```python
from build123d import *

# Parameters (mm, degrees)
F2_R     = 4.064
F3_DEPTH = 12.7
F3_TAPER = 1
F5_DEPTH = 0.79375
F6_COUNT = 8


with BuildPart() as f1:
    # F0 (on Front) → F1 (revolve)
    with BuildSketch(Plane.XZ):
        Polygon((-6.35, 0), (0, 0), (0, 22.9133968065), (-3.175, 22.9133968065), (-3.175, 16.5633968065), (-6.35, 9.525), align=None)
    revolve(axis=Axis((0, 0, 20.1071155777), (0, 0, 1)))

    # F2 (on face) → F3 (join)
    with BuildSketch(Plane(origin=(0, 0, 0), x_dir=(1, 0, 0), z_dir=(0, 0, -1))):
        Circle(F2_R)
    extrude(amount=F3_DEPTH, taper=F3_TAPER)

    # F4 (on Front) → F5 (join, symmetric)
    with BuildSketch(Plane.XZ):
        Polygon((-18.3153760806, 1.7450850807), (-6.35, 0), (-6.0325, 0), (-6.0325, 9.4567020336), (-2.8575, 16.4950988401), (-2.8575, 22.9133968065), (-3.175, 22.9133968065), (-6.35, 22.9133968065), (-38.1, 28.0183404684), (-12.5059876591, 9.994440712), align=None)
    extrude(amount=F5_DEPTH, both=True)

    # F6: F1 ×8 about axis
    f6_axis = Axis((0, 0, 20.1071155777), (0, 0, 1))


with BuildPart() as f1_1:
    add(f1.part)
    for i in range(1, F6_COUNT):
        add(f1.part.rotate(f6_axis, i * 360 / F6_COUNT))


solid = f1_1.part
```
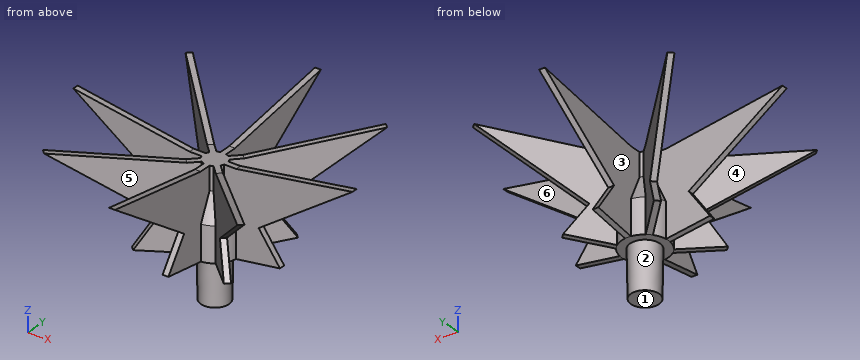
CAD build for the part. Positions are in the model's coordinates, mm. Face numbers are marked on the shaded views. A direction names the side the tool comes from. Coordinates: 2 decimals unless noted, no trailing zeros. Order: outer loops, then holes, each group sorted by start corner. A loop starts at its lowest first (then second) coordinate and runs counter-clockwise, first axis right, second up. Notation, with made-up numbers: (56.5, 57.5) -> (84.5, 57.5) arc R11 ccw to (84.5, 75.5) -> close; hole circle Ø6 at (30, 5). An arc over 180 degrees is marked (long way). Use one line per item in the form item = value. Start each with the question number.
1) Drill centre lines: L1, parallel to X at y = 10.5, z = 3.5; L2, parallel to X at y = 21, z = 19.5; L3, parallel to X at y = -23, z = 26. Where is each one in solid material? Low to high. Write a range as [from, to].
2) Band-saw the part on A-A on y = -14.5. Give the cut face in (x, z), then the cut area to 3 significant figures.
3) Pull direction X, two halves, no side cores. Call the marked faces 3, 4, 5 and 6: +X half, -X half, draft (parallel to the pull), parting line (faces both ways), or undercut.
4) Band-saw the part on C-C on x = 17. Give the cut face in (y, z), then the cut area to 3 significant figures.
5) Band-saw the part on B-B on x = -21.5. Give the cut face in (y, z).
6) Tool access for the marked faces 1 and 2: list every direction of +Z, -Z, +X, -X, +Y, -Y with a clear straight run to the whole face (end or side of a thin tool).
7) Drop flat-ended pins along their axis: pin 1 (22.5 mm diameter, centred on y = 26.5, z = 20.5, fed in from +X); pin 2 (5 mm diameter, centred on x = -8, z = 22.5, fed in from +Y); pin 3 (22.5 mm diameter, centred on x = 23, z = 7.5, fed in from -Y). Give the stop position or say it passes through.
Entries:
q1.L1 = [-11.62, -9.38], [-0.79, 0.79], [9.38, 11.62]
q1.L2 = [-0.79, 0.79]
q1.L3 = [-24.12, -21.88], [21.88, 24.12]
q2.outline = (-15.62, 16.19) -> (-13.38, 15.07) -> (-13.38, 25.06) -> (-15.62, 25.32) -> close; (-0.79, 1.19) -> (0.79, 1.19) -> (0.79, 7.16) -> (-0.79, 7.16) -> close; (-0.79, 11.4) -> (0.79, 11.4) -> (0.79, 24.22) -> (-0.79, 24.22) -> close; (13.38, 15.07) -> (15.62, 16.19) -> (15.62, 25.32) -> (13.38, 25.06) -> close
q2.area = 72.8 mm2
q3.face_3 = undercut
q3.face_4 = -X half
q3.face_5 = undercut
q3.face_6 = draft
q4.outline = (-18.12, 18.68) -> (-15.88, 17.56) -> (-15.88, 25.63) -> (-18.12, 25.89) -> close; (-0.79, 1.55) -> (0.79, 1.55) -> (0.79, 3.61) -> (-0.79, 3.61) -> close; (-0.79, 13.16) -> (0.79, 13.16) -> (0.79, 24.63) -> (-0.79, 24.63) -> close; (15.88, 17.56) -> (18.12, 18.68) -> (18.12, 25.89) -> (15.88, 25.63) -> close
q4.area = 55.8 mm2
q5.outline = (-22.62, 23.16) -> (-20.38, 22.04) -> (-20.38, 26.65) -> (-22.62, 26.91) -> close; (-0.79, 16.33) -> (0.79, 16.33) -> (0.79, 25.35) -> (-0.79, 25.35) -> close; (20.38, 22.04) -> (22.62, 23.16) -> (22.62, 26.91) -> (20.38, 26.65) -> close
q6.face_1 = -Z, +X, -X, +Y, -Y
q6.face_2 = -Z
q7.pin_1 = 27.5
q7.pin_2 = 11.62
q7.pin_3 = -12.57
